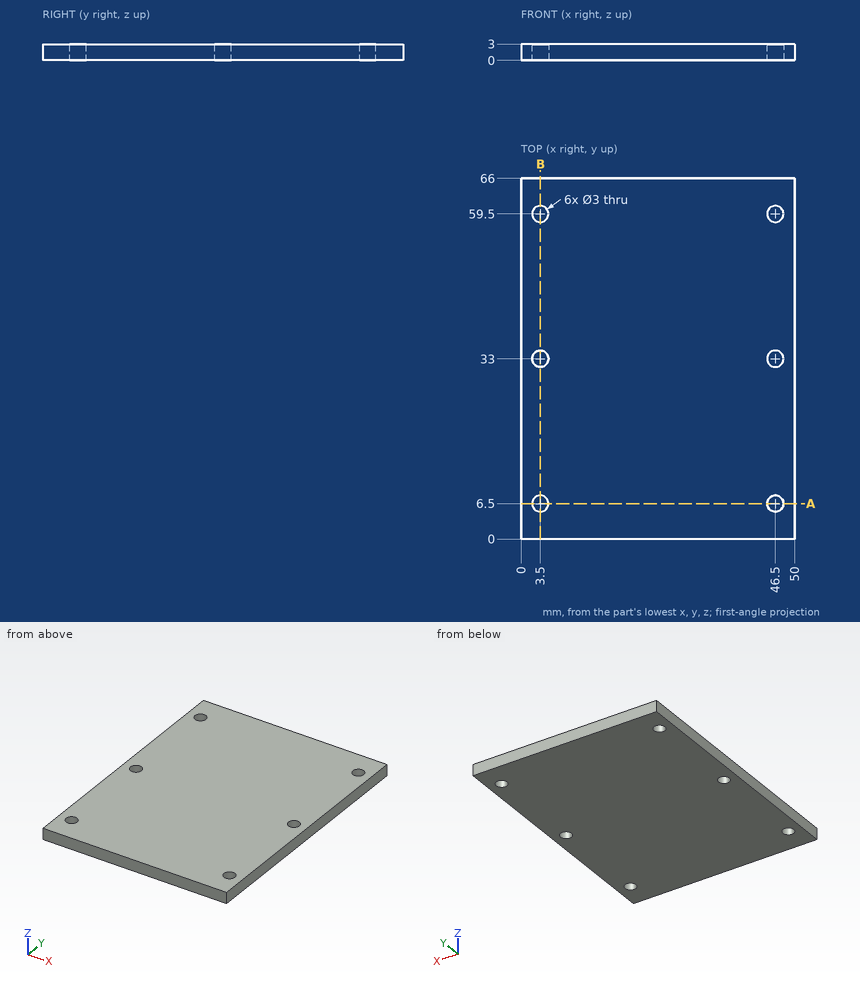
For this review, use the dimensioned drawing (mm, ordinates from the lowest corner) and the shaded views. Round coordinates to 2 decimals unless told otherwise and drop trailing zeros. Write each loop counter-clockwise with the first axis right and the second up, starting at its lowest first coordinate (ties: lowest second). Pieces come first, ordered by that corner, then holes. Notation, with made-up numbers: (-6.75, -39.5) -> (36.25, -39.5) arc R20 ccw to (36.25, -8.5) -> close; hole circle Ø10 at (2, -2.75). An arc over 180 degrees is marked (long way). One line per item, written item: value. Start each with the question number.
Q1. Insertion check: P1, Ø2.5, axis at x = 3.5, y = 6.5, coming from the +Z side. The pin has a flat end and moves straight along its axis. Give the tip position at first contact, or say it passes through.
Q2. To check wall thickness, follow probe 1 along Y at (x, z) = (46.5, 1.2); probe 2 along X at (y, z) = (32, 0.45). State the ranges of each line that lie inside material, in increasing order.
Q3. Add section B-B (x = 3.5). Give the boundary of the cut face in (y, z), then the cut area to 3 significant figures.
Q4. Add section A-A (y = 6.5). Give the boundary of the cut face in (x, z).
Response:
1. P1: passes through
2. probe 1: y = 0 to 5, 8 to 31.5, 34.5 to 58, 61 to 66
2. probe 2: x = 0 to 2.38, 4.62 to 45.38, 47.62 to 50
3. outline: (0, 0) -> (5, 0) -> (5, 3) -> (0, 3) -> close; (8, 0) -> (31.5, 0) -> (31.5, 3) -> (8, 3) -> close; (34.5, 0) -> (58, 0) -> (58, 3) -> (34.5, 3) -> close; (61, 0) -> (66, 0) -> (66, 3) -> (61, 3) -> close
3. area: 171 mm^2
4. outline: (0, 0) -> (2, 0) -> (2, 3) -> (0, 3) -> close; (5, 0) -> (45, 0) -> (45, 3) -> (5, 3) -> close; (48, 0) -> (50, 0) -> (50, 3) -> (48, 3) -> close
